Geometry check sheet. Reference: the model listing, model coordinates, mm. Coordinates: 2 decimals unless noted, no trailing zeros. Put each result on its own line as item: value.
from build123d import *

# Parameters (mm, degrees)
SKETCH1_W            = 270
SKETCH1_H            = 10
BOSS_EXTRUDE1_DEPTH  = 2
CHAMFER1_SIZE        = 2
M3_CLEARANCE_HOLE1_D = 3.4
LPATTERN1_COUNT      = 8
LPATTERN1_PITCH      = 35.714285714


with BuildPart() as part:
    # Sketch1 → Boss-Extrude1 (new body)
    with BuildSketch(Plane.XY):
        Rectangle(SKETCH1_W, SKETCH1_H)
    extrude(amount=BOSS_EXTRUDE1_DEPTH)

    # Chamfer1
    chamfer1_edges = [part.edges().sort_by_distance(p)[0] for p in [
        (135, -5, 1),
        (-135, -5, 1),
    ]]
    chamfer(chamfer1_edges, length=CHAMFER1_SIZE)

    # M3 Clearance Hole1 (through all)
    with Locations(Plane.XY.offset(2)):
        with Locations((125, 0)):
            m3_clearance_hole1 = Hole(M3_CLEARANCE_HOLE1_D / 2)

    # LPattern1: M3 Clearance Hole1 ×8
    with Locations(*[(-i * LPATTERN1_PITCH, 0, 0) for i in range(1, LPATTERN1_COUNT)]):
        add(m3_clearance_hole1, mode=Mode.SUBTRACT)


solid = part.part
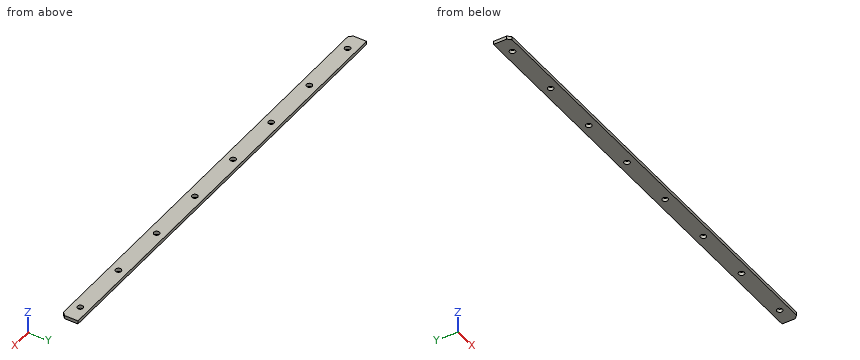
Q1. Depth check by flat-ended pin: pin 1 Ø4 at (x, y) = (-125, 0) entering from -Z. Enter the tip coordinate at first touch or a pass-through.
Answer block:
pin 1: stops at z = 0
Q2. Section check A-A on z = 0.4. State how many separate pieces and enclosed holes the cut face has, then the cut area to 3 significant figures.
Answer block:
separate pieces: 1
enclosed holes: 8
area: 2,620 mm^2
Q3. Thickness scan on L1, parallel to Y at x = 18, z = 0.3; L2, parallel to X at y = -3.25, z = 1.9. Record the ranges inside material, lowest first. Write a range as [from, to].
Answer block:
L1: y = [-5, -1.69], [1.69, 5]
L2: x = [-134.75, 134.75]
